Geometry: final body of the model. Coordinates: model frame, mm. Give positions to 0.01 mm unless a question says otherwise; leave off trailing zeros. Write each loop counter-clockwise with the first axis right and the second up, starting at its lowest first coordinate (ties: lowest second). Pieces come first, ordered by that corner, then holes.
Q1. Cut plane C-C on x = -51. Return the cut outline in (y, z), plus the area to 3 significant figures.
Q2. Pin query (flat end, axial travel): pin 1 (2.5 mm diameter, centred on x = -143.45, z = 5, fed in from +Y); pin 2 (5 mm diameter, centred on x = -36.55, z = 5, fed in from +Y); pin 3 (1.5 mm diameter, centred on y = 10, z = 5.5, fed in from -X). Return the tip coordinate at first contact, or that it passes through.
Q3. Line query: L1, parallel to Z at x = -95, y = 8.5; L2, parallel to Z at x = -36.55, y = 2.5; L3, parallel to Y at x = -84, z = 7. Output: solid intervals per line, ascending.
Q4. Cut plane A-A on x = -153.45. Return the cut outline in (y, z), plus the area to 3 significant figures.
Q5. Cut plane B-B on y = 4.5. Count the separate pieces of the cut face and the enclosed holes in it, plus the area to 3 significant figures.
Q6. Draft query along Z for faces 1 (the face through (20, 5, 5)), 2 (the face through (-10, 13, 5)), 3 (the face through (-165.698, 5.07, 4.901)). Return one class per face: pulls with the +Z half, pulls with the -Z half, needs draft (parallel to the pull), parting line crosses it, or undercut.
Autodesk Inventor part; units mm, degrees
ref_plane "YZ Plane" through (0, 0, 0) normal (1, 0, 0) x (0, 1, 0)
ref_plane "XZ Plane" through (0, 0, 0) normal (0, 1, 0) x (-1, 0, 0)
ref_plane "XY Plane" through (0, 0, 0) normal (0, 0, 1) x (1, 0, 0)
sketch "Sketch1" plane through (0, 0, 0) normal (0, 1, 0) x (-1, 0, 0)
  line L0 (0, 0) -> (170, 0)
  line L1 (170, 0) -> (170, 10)
  line L2 (170, 10) -> (0, 10)
  line L3 (0, 10) -> (0, 0)
  dimension "d0" = 170
  dimension "d1" = 10
extrude "Extrusion1" add sketch "Sketch1" along normal blind 10
sketch "Sketch2" plane through (0, 10, 0) normal (0, 1, 0) x (1, 0, 0)
  line L0 (0, -10) -> (0, 0)
  line L1 (0, -5) -> (-2.2, -5)
  circle A0 centre (-6.1, -5) radius 3.9
  line L2 (0, 0) -> (-170, 0)
  line L3 (-170, -10) -> (0, -10)
  circle A1 centre (-75, -5) radius 1.5
  circle A2 centre (-95, -5) radius 1.5
  dimension "d35" = 10
  dimension "d4" = 2.2
  dimension "d8" = 3
  dimension "d9" = 3
extrude "Extrusion2" cut sketch "Sketch2" against normal blind 10 contours A1
extrude "Extrusion3" cut sketch "Sketch2" against normal blind 10 contours A2
extrude "Extrusion4" add sketch "Sketch2" along normal blind 7 contours A0
sketch "Sketch3" plane through (0, 10, 0) normal (0, 1, 0) x (1, 0, 0)
  line L0 (-170, 0) -> (-170, -10)
  line L1 (-170, -5) -> (-10, -5)
  circle A0 centre (-6.1, -5) radius 3.9
  line L2 (-165.7, -5) -> (-163.45, -5)
  circle A1 centre (-163.45, -5) radius 2.25
  circle A2 centre (-153.45, -5) radius 2.25
  circle A3 centre (-143.45, -5) radius 2.25
  circle A4 centre (-133.45, -5) radius 2.25
  circle A5 centre (-123.45, -5) radius 2.25
  circle A6 centre (-113.45, -5) radius 2.25
  circle A7 centre (-103.45, -5) radius 2.25
  circle A8 centre (-95, -5) radius 1.5
  line L3 (-93.5, -5) -> (-93.5, -7.9104)
  circle A9 centre (-75, -5) radius 1.5
  line L4 (-76.5, -5) -> (-76.5, -7.25)
  line L5 (-93.5, -5) -> (-76.5, -5)
  line L6 (-85, -5) -> (-93.5, -5)
  line L7 (-85, -5) -> (-76.5, -5)
  circle A10 centre (-80.75, -5) radius 2.25
  circle A11 centre (-89.25, -5) radius 2.25
  line L8 (-10, -5) -> (-12, -5)
  line L9 (-10, -5) -> (-14.3, -5)
  line L10 (-14.3, -5) -> (-16.55, -5)
  circle A12 centre (-16.55, -5) radius 2.25
  circle A13 centre (-26.55, -5) radius 2.25
  circle A14 centre (-36.55, -5) radius 2.25
  circle A15 centre (-46.55, -5) radius 2.25
  circle A16 centre (-56.55, -5) radius 2.25
  circle A17 centre (-66.55, -5) radius 2.25
  point P0 (0, 0)
  point P1 (-155.7, -5)
  point P2 (-145.7, -5)
  point P3 (-135.7, -5)
  point P4 (-125.7, -5)
  point P5 (-115.7, -5)
  point P6 (-105.7, -5)
  point P7 (-24.3, -5)
  point P8 (-34.3, -5)
  point P9 (-44.3, -5)
  point P10 (-54.3, -5)
  point P11 (-64.3, -5)
  dimension "d20" = 10
  dimension "d32" = 10
extrude "Extrusion5" cut sketch "Sketch3" against normal blind 10 contours A1 L1 | L1 A1 | L1 A12 | L1 A12 | A2 L1 | L1 A2 | A3 L1 | L1 A3 | A4 L1 | L1 A4 | A5 L1 | L1 A5 | A6 L1 | L1 A6 | A7 L1 | L1 A7 | A11 L1 | L1 A11 | A10 L1 | L1 A10 | A17 L1 | L1 A17 | A16 L1 | L1 A16 | A15 L1 | L1 A15 | A14 L1 | L1 A14 | A13 L1 | L1 A13
thread "Thread1"
thread "Thread2"
sketch "Sketch4" plane through (0, 10, 0) normal (0, 1, 0) x (1, 0, 0)
  circle A0 centre (-16.55, -5) radius 2.25
  circle A1 centre (-16.55, -5) radius 2.25
  point P0 (0, 0)
extrude "Extrusion6" add sketch "Sketch4" against normal blind 10
sketch "Sketch5" plane through (0, 0, 10) normal (1, 0, 0) x (0, 0, -1)
  line L0 (10, 0) -> (0, 0)
  line L1 (0, 0) -> (0, 10)
  line L2 (10, 0) -> (0, 0)
  line L3 (0, 0) -> (0, 10)
  line L4 (0, 10) -> (10, 10)
  line L5 (10, 10) -> (10, 0)
extrude "Extrusion7" add sketch "Sketch5" along normal blind 10
sketch "Sketch6" plane through (10, 0, 10) normal (1, 0, 0) x (0, 0, -1)
  line L0 (0, 0) -> (10, 0)
  line L1 (0, 10) -> (0, 0)
  line L2 (10, 0) -> (0, 0)
  line L3 (0, 0) -> (0, 10)
  line L4 (0, 10) -> (10, 10)
  line L5 (10, 10) -> (10, 0)
extrude "Extrusion8" add sketch "Sketch6" along normal blind 10
sketch "Sketch7" plane through (0, 10, 0) normal (0, 1, 0) x (1, 0, 0)
  point P0 (0, 0)
fillet "Fillet3" radius 1 11 edges at (-75, 10, 10) (-75, 0, 10) (-75, 10, 0) (20, 5, 10) (20, 5, 0) (20, 0, 5) (-170, 10, 5) (-170, 5, 10) (-170, 5, 0) (-170, 0, 5) (-75, 0, 0)
fillet "Fillet4" radius 1 3 edges at (19.7071, 9.7071, 9.7071) (19.7071, 9.7071, 0.2929) (20, 10, 5)
properties part number "brazo apoyo"
Data:
1. outline: (0, 1) arc R1 ccw to (1, 0) - (9, 0) arc R1 ccw to (10, 1) - (10, 9) arc R1 ccw to (9, 10) - (1, 10) arc R1 ccw to (0, 9) - close
1. area: 99.1 mm2
2. pin 1: passes through
2. pin 2: stops at y = 10
2. pin 3: stops at x = -169.97
3. L1: z = 0 to 3.5, 6.5 to 10
3. L2: z = 0 to 2.75, 7.25 to 10
3. L3: y = 0 to 10
4. outline: (0, 1) arc R1 ccw to (1, 0) - (9, 0) arc R1 ccw to (10, 1) - (10, 2.75) - (0, 2.75) - close; (0, 7.25) - (10, 7.25) - (10, 9) arc R1 ccw to (9, 10) - (1, 10) arc R1 ccw to (0, 9) - close
4. area: 54.1 mm2
5. separate pieces: 1
5. enclosed holes: 16
5. area: 1,660 mm2
6. face 1: needs draft
6. face 2: parting line crosses it
6. face 3: undercut
